from build123d import *

# Parameters (mm, degrees)
SCHIZZO1_R                   = 12
SCHIZZO1_R_2                 = 10
ESTRUSIONE_ESTRUSIONE1_DEPTH = 34
SMUSSO1_SIZE                 = 0.3


with BuildPart() as part:
    # Schizzo1 → Estrusione-Estrusione1 (new body)
    with BuildSketch(Plane.XY):
        Circle(SCHIZZO1_R)
        Circle(SCHIZZO1_R_2, mode=Mode.SUBTRACT)
    extrude(amount=ESTRUSIONE_ESTRUSIONE1_DEPTH)

    # Smusso1
    smusso1_edges = [part.edges().sort_by_distance(p)[0] for p in [
        (-12, 0, 0),
        (-12, 0, 34),
        (-10, 0, 0),
        (-10, 0, 34),
    ]]
    chamfer(smusso1_edges, length=SMUSSO1_SIZE)


solid = part.part
Geometry: final body of the model. Coordinates: model frame, mm. Coordinates: 2 decimals unless noted, no trailing zeros. Order: outer loops, then holes, each group sorted by start corner. A loop starts at its lowest first (then second) coordinate and runs counter-clockwise, first axis right, second up.
(1) Section query A-A (y = 0). Return the cut outline in (x, z), plus the area to 3 significant figures.
(2) Section query C-C (z = 27). Return the cut outline in (x, y).
(3) Material intervals for probe 1 along Y at (x, z) = (0, 24); probe 2 along Y at (x, z) = (1, 11.5); probe 3 along X at (y, z) = (6.75, 31.5), sorted ascending.
(4) Draft query along X for faces 1 (the face through (-11.99, 0.53, 16.77)), 2 (the face through (7, -8, 34)), 3 (the face through (-2.17, -9.76, 16.77)). Return one class per face: pulls with the +X half, pulls with the -X half, needs draft (parallel to the pull), parting line crosses it, or undercut.
(5) First-contact query: pin 1 (8 mm diameter, centred on x = 7, z = 11.5, fed in from +Y); pin 2 (1 mm diameter, centred on y = 8.5, z = 17.5, fed in from +X); pin 3 (1 mm diameter, centred on x = 7.5, y = -4, fed in from +Z); pin 4 (10 mm diameter, centred on x = -7, z = 23.5, fed in from -Y). Flat tips, straight axial feed; report the tip coordinate or a pass-through.
Solution:
1. outline: (-12, 0.3) - (-11.7, 0) - (-10.3, 0) - (-10, 0.3) - (-10, 33.7) - (-10.3, 34) - (-11.7, 34) - (-12, 33.7) - close; (10, 0.3) - (10.3, 0) - (11.7, 0) - (12, 0.3) - (12, 33.7) - (11.7, 34) - (10.3, 34) - (10, 33.7) - close
1. area: 136 mm2
2. outline: circle Ø24 at (0, 0); hole circle Ø20 at (0, 0)
3. probe 1: y = -12 to -10, 10 to 12
3. probe 2: y = -11.96 to -9.95, 9.95 to 11.96
3. probe 3: x = -9.92 to -7.38, 7.38 to 9.92
4. face 1: parting line crosses it
4. face 2: needs draft
4. face 3: undercut
5. pin 1: stops at y = 11.62
5. pin 2: stops at x = 8.94
5. pin 3: passes through
5. pin 4: stops at y = -11.83
